Verification items for this drawing (mm, ordinates from the low corner). A direction names the side the tool comes from. Give positions to 0.01 mm unless a question says otherwise; leave off trailing zeros. Order: outer loops, then holes, each group sorted by start corner. A loop starts at its lowest first (then second) coordinate and runs counter-clockwise, first axis right, second up. Notation, with made-up numbers: (79, -26.75) -> (117, -26.75) arc R5 cw to (117, -22.75) -> close; hole circle Ø9 at (36.25, 69.5). An arc over 180 degrees is marked (long way). One line per question, with ' | ' between items.
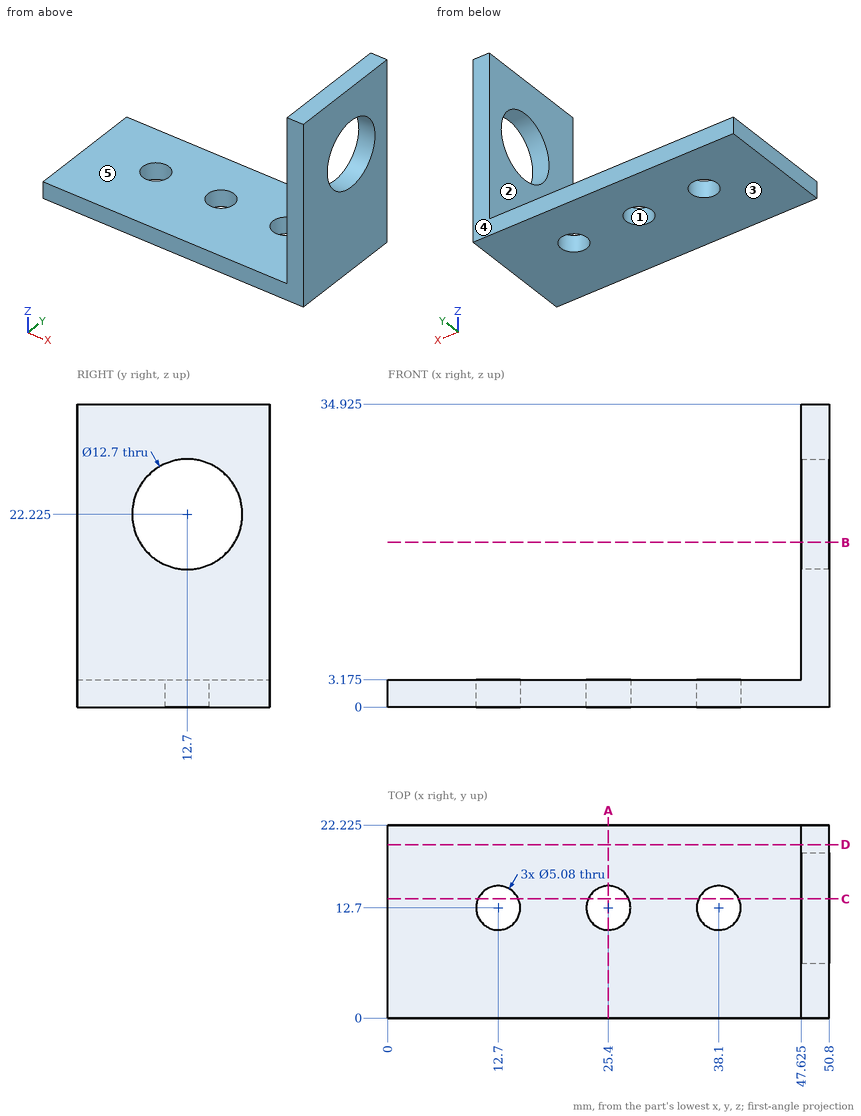
Q1. Thickness scan on line 1 (Y direction, x = 12.7, z = 1.3) (3 decimals); line 2 (Z direction, x = 15, y = 19.25) (3 decimals); line 3 (X direction, y = 13.5, z = 30) (3 decimals). Record the ranges inside material, lowest first.
Result sheet:
line 1: y = 0 to 10.16, 15.24 to 22.225 | line 2: z = 0 to 3.175 | line 3: x = 47.625 to 50.8
Q2. Section check B-B (z = 19). Enter the section's corners in (x, y) (3 decimals).
Result sheet:
outline: (47.625, 0) -> (50.8, 0) -> (50.8, 7.23) -> (47.625, 7.23) -> close; (47.625, 18.17) -> (50.8, 18.17) -> (50.8, 22.225) -> (47.625, 22.225) -> close
Q3. Section check D-D (y = 20). Enter the section's corners in (x, z) (3 decimals), and give its area (3 significant figures).
Result sheet:
outline: (0, 0) -> (50.8, 0) -> (50.8, 34.925) -> (47.625, 34.925) -> (47.625, 3.175) -> (0, 3.175) -> close | area: 262 mm2
Q4. Access from +Z, -Z, +X, -X, +Y, -Y to the whole of each face (thin tool, end or side, straight path). Record for the marked faces 4 and 5.
Result sheet:
face 4: +Z, -Z, +X, -X, +Y | face 5: +Z, -X, +Y, -Y
Q5. Mould release check, pull along X, two halves, no side actions. Record for the marked faces 1, 2 and 3: pulls with the +X half, pulls with the -X half, needs draft (parallel to the pull), parting line crosses it, or undercut.
Result sheet:
face 1: undercut | face 2: pulls with the -X half | face 3: needs draft
Q6. Section check A-A (x = 25.4). Enter the section's corners in (y, z) (3 decimals), and give its area (3 significant figures).
Result sheet:
outline: (0, 0) -> (10.16, 0) -> (10.16, 3.175) -> (0, 3.175) -> close; (15.24, 0) -> (22.225, 0) -> (22.225, 3.175) -> (15.24, 3.175) -> close | area: 54.4 mm2
Q7. Section check C-C (y = 13.75). Enter the section's corners in (x, z) (3 decimals).
Result sheet:
outline: (0, 0) -> (10.387, 0) -> (10.387, 3.175) -> (0, 3.175) -> close; (15.013, 0) -> (23.087, 0) -> (23.087, 3.175) -> (15.013, 3.175) -> close; (27.713, 0) -> (35.787, 0) -> (35.787, 3.175) -> (27.713, 3.175) -> close; (40.413, 0) -> (50.8, 0) -> (50.8, 15.962) -> (47.625, 15.962) -> (47.625, 3.175) -> (40.413, 3.175) -> close; (47.625, 28.488) -> (50.8, 28.488) -> (50.8, 34.925) -> (47.625, 34.925) -> close
Q8. Depth check by flat-ended pin: pin 1 Ø8 at (x, y) = (38.1, 12.7) entering from +Z (3 decimals); pin 2 Ø4 at (y, z) = (8, 27) entering from -X (3 decimals). Enter the tip coordinate at first touch or a pass-through.
Result sheet:
pin 1: stops at z = 3.175 | pin 2: stops at x = 47.625
